```python
from build123d import *

# Parameters (mm, degrees)
F0_W          = 598.4875
F0_H          = 170.18
F1_DEPTH      = 2.794
F2_W          = 5.588
F2_H          = 170.18
F3_DEPTH      = 419.1
F4_W          = 587.3115
F4_H          = 5.588
F5_DEPTH      = 413.512
F6_W          = 19.05
F6_H          = 9.525
F7_DEPTH      = 598.4885
F8_R          = 3.175
F9_DEPTH      = 5.589
F9_DEPTH_BACK = 592.9005


with BuildPart() as f1:
    # F0 (on Front) → F1 (new body, symmetric)
    with BuildSketch(Plane.XZ):
        Rectangle(F0_W, F0_H)
    extrude(amount=F1_DEPTH, both=True)

    # F2 (on face) → F3 (join)
    with BuildSketch(Plane.XZ.offset(2.794)):
        with Locations((-296.44975, 0)):
            Rectangle(F2_W, F2_H)
        with Locations((296.44975, 0)):
            Rectangle(F2_W, F2_H)
    extrude(amount=-F3_DEPTH)

    # F4 (on face) → F5 (join, through all)
    with BuildSketch(Plane(origin=(0, 2.794, 0), x_dir=(-1, 0, 0), z_dir=(0, 1, 0))):
        with Locations((0, -82.296)):
            Rectangle(F4_W, F4_H)
    extrude(amount=F5_DEPTH)

    # F6 (on face) → F7 (cut, through all)
    with BuildSketch(Plane.YZ.offset(299.24375)):
        with Locations((406.781, 80.3275)):
            Rectangle(F6_W, F6_H)
    extrude(amount=-F7_DEPTH, mode=Mode.SUBTRACT)

    # F8 (on face) → F9 (cut, two sides)
    with BuildSketch(Plane.YZ.offset(-293.65575)) as f9_sk:
        with Locations((403.606, 62.865)):
            Circle(F8_R)
        with Locations((333.756, 62.865)):
            Circle(F8_R)
        with Locations((16.256, 62.865)):
            Circle(F8_R)
    extrude(amount=-F9_DEPTH, mode=Mode.SUBTRACT)
    extrude(f9_sk.sketch, amount=F9_DEPTH_BACK, mode=Mode.SUBTRACT)


solid = f1.part
```
Source: CAD feature listing. Evaluate the final solid. Frame: model axes, mm. A direction names the side the tool comes from. Coordinates: 2 decimals unless noted, no trailing zeros. Loops run counter-clockwise (first coordinate to the right, second up) from the corner with the lowest first, then second, coordinate; pieces in that order, holes last. Notation, with made-up numbers: (71.25, 24) -> (119.25, 24) arc R24 cw to (119.25, 48) -> close; hole circle Ø1 at (-18, 48). An arc over 180 degrees is marked (long way). One line per item, written item: value. Start each with the question number.
Q1. Section query A-A, the plane z = 46.5. Return the cut outline in (x, y), and give its area (3 significant figures).
Q2. Section query C-C, the plane x = -173. Return the cut outline in (y, z), and give its area (3 significant figures).
Q3. Section query B-B, the plane y = 34. Return the cut outline in (x, z).
Q4. Contact query for flat-ended pins moving along their axis: P1, Ø10, axis at x = 75.5, y = 165, coming from the +Z side; P2, Ø3, axis at x = -297, y = 403.5, coming from the +Z side (3 decimals); P3, Ø2, axis at x = 179, z = -47.5, coming from the +Y side. Output: stop coordinate, or through.
Q5. Set-up query: faces 1 (the face through (293.656, 207, 2)), 2 (the face through (1, 416.306, -82)). Return all of +Z, -Z, +X, -X, +Y, -Y with unobstructed straight access to the full face (end or side cutting, diameter ignored); none if empty.
Q6. Line query: line 1 along X through (y, z) = (389, 22); line 2 along Z through (x, y) = (-124, 309.5); line 3 along Y through (x, z) = (-210.5, 64.5). Output: solid intervals per line, ascending.
Results:
1. outline: (-299.24, -2.79) -> (299.24, -2.79) -> (299.24, 416.31) -> (293.66, 416.31) -> (293.66, 2.79) -> (-293.66, 2.79) -> (-293.66, 416.31) -> (-299.24, 416.31) -> close
1. area: 7,970 mm^2
2. outline: (-2.79, -85.09) -> (416.31, -85.09) -> (416.31, -79.5) -> (2.79, -79.5) -> (2.79, 85.09) -> (-2.79, 85.09) -> close
2. area: 3,260 mm^2
3. outline: (-299.24, -85.09) -> (299.24, -85.09) -> (299.24, 85.09) -> (293.66, 85.09) -> (293.66, -79.5) -> (-293.66, -79.5) -> (-293.66, 85.09) -> (-299.24, 85.09) -> close
4. P1: z = -79.5
4. P2: z = 75.565
4. P3: y = 2.79
5. face 1: +Z, +Y
5. face 2: +Z, -Z, +X, -X, +Y
6. line 1: -299.24 to -293.66, 293.66 to 299.24
6. line 2: -85.09 to -79.5
6. line 3: -2.79 to 2.79
